Job drawing, mm, ordinate dimensions from the low corner. One solid piece. A direction names the side the tool comes from. Coordinates: 2 decimals unless noted, no trailing zeros. Loops run counter-clockwise (first coordinate to the right, second up) from the corner with the lowest first, then second, coordinate; pieces in that order, holes last. Notation, with made-up numbers: (66, 76.5) - (113, 76.5) arc R11 ccw to (113, 91.5) - close; hole circle Ø1 at (-14, 7.25). An arc over 180 degrees is marked (long way). Use a Markdown table: item, result. Add a question column.
1. Pull direction Z, two halves, no side cores. Call the marked faces 1, 2 and 3: pulls with the +Z half, pulls with the -Z half, needs draft (parallel to the pull), parting line crosses it, or undercut.
2. Drop flat-ended pins along their axis: pin 1 (6.5 mm diameter, centred on y = 4, z = 9.5, fed in from -X); pin 2 (23.5 mm diameter, centred on x = 32, z = 41.5, fed in from -Y); pin 3 (1.8 mm diameter, centred on x = 21.5, y = 3.5, fed in from +Z); pin 4 (6.5 mm diameter, centred on x = 52.5, y = 2.5, fed in from +Z). Give the stop position or say it passes through.
3. Band-saw the part on A-A, the plane x = 67.05. Give the cut face in (y, z) (3 decimals), plus the area to 3 significant figures.
4. Wall check: probe 1 along Y at (x, z) = (21.35, 4.25); probe 2 along X at (y, z) = (3, 68.55) (3 decimals); probe 3 along Z at (x, y) = (67.05, 16.5) (3 decimals). Give the ranges that are in metal, low to high. Write a range as [from, to].
5. Band-saw the part on B-B, the plane z = 29.15. Give the cut face in (x, y) (3 decimals).
6. Band-saw the part on D-D, the plane x = 24. Give the cut face in (y, z), plus the area to 3 significant figures.
7. Band-saw the part on C-C, the plane y = 3. Count the separate pieces of the cut face and the enclosed holes in it, plus the area to 3 significant figures.
8. 3-axis set-ups, long thin cutter, end or side, ignore diameter. For the marked faces 4 and 5: which of +Z, -Z, +X, -X, +Y, -Y reach the whole face in a straight line?
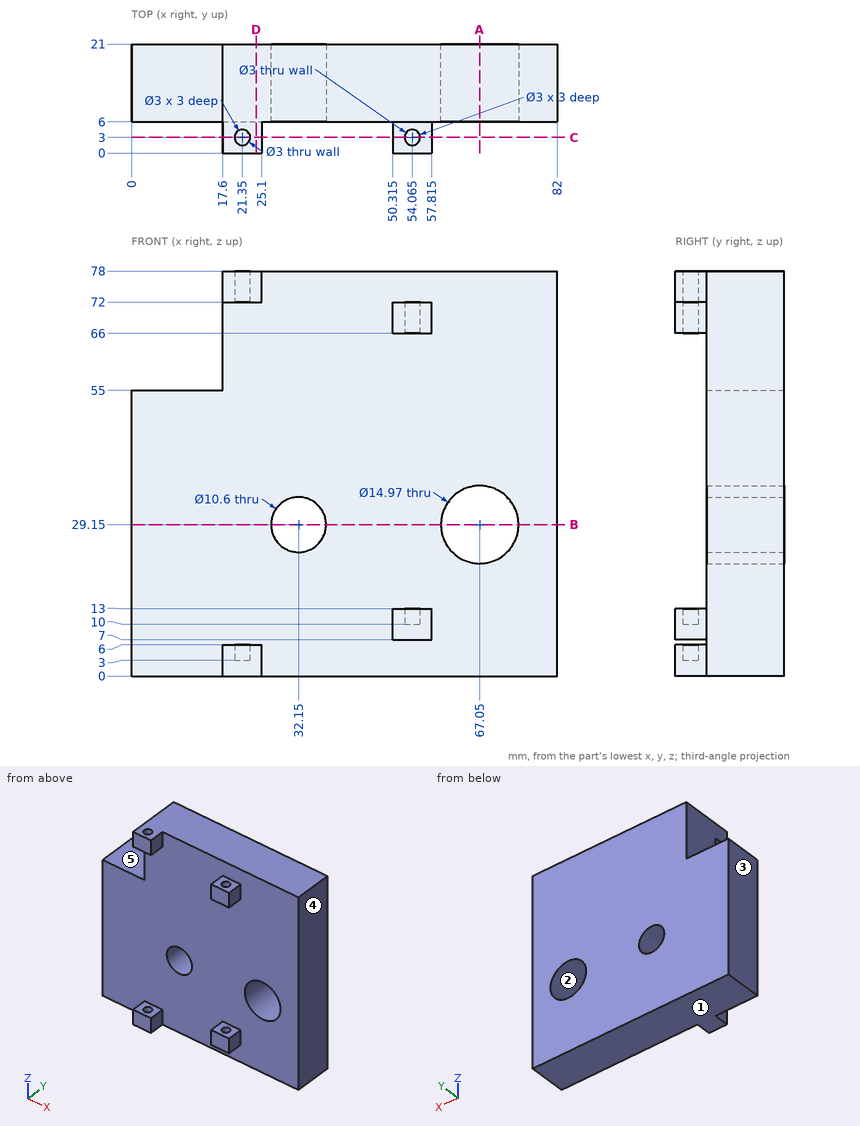
Geometry check:
| question | item | result |
|---|---|---|
| 1 | face 1 | pulls with the -Z half |
| 1 | face 2 | undercut |
| 1 | face 3 | needs draft |
| 2 | pin 1 | stops at x = 0 |
| 2 | pin 2 | stops at y = 6 |
| 2 | pin 3 | stops at z = 3 |
| 2 | pin 4 | stops at z = 72 |
| 3 | outline | (6, 0) - (21, 0) - (21, 21.665) - (6, 21.665) - close; (6, 36.635) - (21, 36.635) - (21, 78) - (6, 78) - close |
| 3 | area | 945 mm^2 |
| 4 | probe 1 | y = [0, 1.5], [4.5, 21] |
| 4 | probe 2 | x = [50.315, 52.565], [55.565, 57.815] |
| 4 | probe 3 | z = [0, 21.665], [36.635, 78] |
| 5 | outline | (0, 6) - (26.85, 6) - (26.85, 21) - (0, 21) - close; (37.45, 6) - (59.565, 6) - (59.565, 21) - (37.45, 21) - close; (74.535, 6) - (82, 6) - (82, 21) - (74.535, 21) - close |
| 6 | outline | (0, 0) - (21, 0) - (21, 78) - (0, 78) - (0, 72) - (6, 72) - (6, 6) - (0, 6) - close |
| 6 | area | 1,240 mm^2 |
| 7 | separate pieces | 6 |
| 7 | enclosed holes | 0 |
| 7 | area | 126 mm^2 |
| 8 | face 4 | +Z, -Z, +X, +Y, -Y |
| 8 | face 5 | +Z, -X, +Y, -Y |
